Geometry check sheet. Reference: the model listing, model coordinates, mm. Face numbers are marked on the shaded views. A direction names the side the tool comes from. Give positions to 0.01 mm unless a question says otherwise; leave off trailing zeros. Loops run counter-clockwise (first coordinate to the right, second up) from the corner with the lowest first, then second, coordinate; pieces in that order, holes last. Notation, with made-up numbers: (20, 19) - (51, 19) arc R16 ccw to (51, 39) - close; hole circle Ø1 at (31.5, 2). An arc over 180 degrees is marked (long way). One line per question, with ' | ' between items. Start each with the question number.
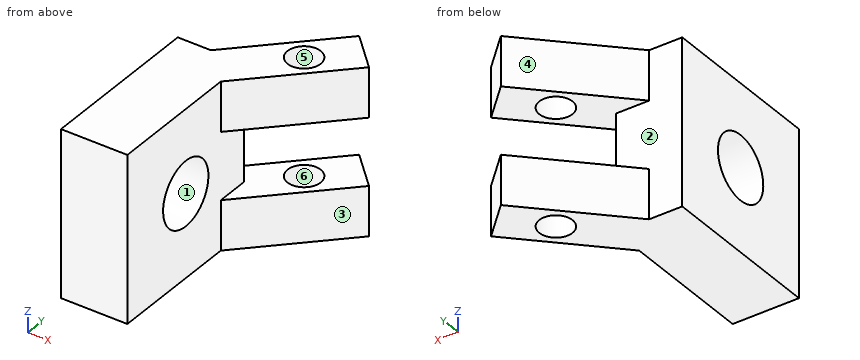
from build123d import *

# Parameters (mm, degrees)
SKETCH1_W           = 25
SKETCH1_H           = 25
SKETCH1_R           = 4.85
BOSS_EXTRUDE1_DEPTH = 10
BOSS_EXTRUDE2_DEPTH = 12.5
CUT_EXTRUDE1_DEPTH  = 5.05
SKETCH4_R           = 2.5
CUT_EXTRUDE2_DEPTH  = 43.598275722
SCALE1_SCALE        = 1.5


with BuildPart() as part:
    # Sketch1 → Boss-Extrude1 (new body)
    with BuildSketch(Plane(origin=(0, 0, 0), x_dir=(0, 0, -1), z_dir=(1, 0, 0))):
        Rectangle(SKETCH1_W, SKETCH1_H)
        Circle(SKETCH1_R, mode=Mode.SUBTRACT)
    extrude(amount=BOSS_EXTRUDE1_DEPTH)

    # Sketch2 → Boss-Extrude2 (add, symmetric)
    with BuildSketch(Plane.XY):
        Polygon((5, 12.5), (18.106601718, 25.606601718), (23.106601718, 20.606601718), (10, 7.5), (10, 12.5), align=None)
    extrude(amount=BOSS_EXTRUDE2_DEPTH, both=True)

    # Sketch3 → Cut-Extrude1 (cut, symmetric)
    with BuildSketch(Plane.XY):
        Polygon((23.106601718, 20.606601718), (18.106601718, 25.606601718), (5, 12.5), (10, 12.5), (10, 7.5), align=None)
    extrude(amount=CUT_EXTRUDE1_DEPTH, both=True, mode=Mode.SUBTRACT)

    # Sketch4 → Cut-Extrude2 (cut, through all)
    with BuildSketch(Plane(origin=(0, 0, -12.5), x_dir=(-1, 0, 0), z_dir=(0, 0, -1))):
        with Locations(Location((-15.303300859, 17.803300859, 0), (0, 0, 90))):
            Circle(SKETCH4_R)
    extrude(amount=-CUT_EXTRUDE2_DEPTH, mode=Mode.SUBTRACT)


with BuildPart() as part_1:
    # Scale1: scaled about (7.010691975, 3.593426571, 0)
    add(part.part.scale(SCALE1_SCALE).moved(Location((-3.505345988, -1.796713286, 0))))


solid = part_1.part
(1) Section check A-A, the plane z = 0. Record the boundary of the cut face in (x, y).
(2) Depth check by flat-ended pin: pin 1 Ø3 at (x, z) = (23, 10.5) entering from +Y; pin 2 Ø12 at (y, z) = (29.5, -0.5) entering from +X; pin 3 Ø7.5 at (x, z) = (5.5, 7.5) entering from +Y. Enter the tip coordinate at first touch or a pass-through.
(3) Section check B-B, the plane y = -7. Record the boundary of the cut face in (x, z).
(4) Mould release check, pull along Y, two halves, no side actions. Record for the marked faces 3, 4, 5 and 6: pulls with the +Y half, pulls with the -Y half, needs draft (parallel to the pull), parting line crosses it, or undercut.
(5) Section check D-D, the plane y = 16. Record the boundary of the cut face in (x, z) (3 decimals).
(6) Section check C-C, the plane x = 18.5. Record the boundary of the cut face in (y, z) (3 decimals), and give its area (3 significant figures).
(7) Tool access check on the marked faces 1 and 2. Record the directions out of +Z, -Z, +X, -X, +Y, -Y that give a thin tool (end or side, any length) a straight path to the whole face; none if there is none.
(8) Material ranges on line 1 (Z direction, x = 15, y = 17.5) (3 decimals); line 2 (Y direction, x = 4, z = 0); line 3 (Y direction, x = 21, z = 15), recorded low to high.
Numbers:
1) outline: (-3.51, -20.55) - (11.49, -20.55) - (11.49, -9.07) - (-3.51, -9.07) - close; (-3.51, 5.48) - (11.49, 5.48) - (11.49, 16.95) - (-3.51, 16.95) - close
2) pin 1: y = 36.61 | pin 2: through | pin 3: y = 22.21
3) outline: (-3.51, -18.75) - (11.49, -18.75) - (11.49, -5.08) - (-3.51, -5.08) - close; (-3.51, 5.08) - (11.49, 5.08) - (11.49, 18.75) - (-3.51, 18.75) - close
4) face 3: pulls with the -Y half | face 4: pulls with the +Y half | face 5: undercut | face 6: undercut
5) outline: (-3.505, -18.75) - (18.041, -18.75) - (18.041, -7.575) - (11.495, -7.575) - (11.495, 7.575) - (18.041, 7.575) - (18.041, 18.75) - (-3.505, 18.75) - close
6) outline: (16.459, -18.75) - (21.28, -18.75) - (21.28, -7.575) - (16.459, -7.575) - close; (16.459, 7.575) - (21.28, 7.575) - (21.28, 18.75) - (16.459, 18.75) - close; (28.536, -18.75) - (31.459, -18.75) - (31.459, -7.575) - (28.536, -7.575) - close; (28.536, 7.575) - (31.459, 7.575) - (31.459, 18.75) - (28.536, 18.75) - close | area: 173 mm^2
7) face 1: +X, -X | face 2: -X, +Y
8) line 1: -18.75 to -7.575, 7.575 to 18.75 | line 2: -20.55 to -9.07, 5.48 to 16.95 | line 3: 18.96 to 21.49, 28.32 to 33.96
